```python
from build123d import *

# Parameters (mm, degrees)
SKETCH1_R           = 5
BOSS_EXTRUDE1_DEPTH = 150
SKETCH2_R           = 5
SKETCH2_R_2         = 4.8
CUT_EXTRUDE1_DEPTH  = 1.15
SKETCH3_R           = 5
SKETCH3_R_2         = 4.8
CUT_EXTRUDE2_DEPTH  = 1.15


with BuildPart() as part:
    # Sketch1 → Boss-Extrude1 (new, symmetric)
    with BuildSketch(Plane.XY):
        Circle(SKETCH1_R)
    extrude(amount=BOSS_EXTRUDE1_DEPTH, both=True)

    # Sketch2 → Cut-Extrude1 (cut)
    with BuildSketch(Plane.XY.offset(148)):
        Circle(SKETCH2_R)
        Circle(SKETCH2_R_2, mode=Mode.SUBTRACT)
    cut_extrude1 = extrude(amount=CUT_EXTRUDE1_DEPTH, mode=Mode.SUBTRACT)

    # Sketch3 → Cut-Extrude2 (cut)
    with BuildSketch(Plane.XY.offset(97.5)):
        Circle(SKETCH3_R)
        Circle(SKETCH3_R_2, mode=Mode.SUBTRACT)
    cut_extrude2 = extrude(amount=-CUT_EXTRUDE2_DEPTH, mode=Mode.SUBTRACT)

    # Mirror1: Cut-Extrude1, Cut-Extrude2 across plane
    add(cut_extrude1.mirror(Plane.XY), mode=Mode.SUBTRACT)
    add(cut_extrude2.mirror(Plane.XY), mode=Mode.SUBTRACT)


solid = part.part
```
The model under review builds one solid part; all positions refer to its coordinate system, in mm. A direction names the side the tool comes from. Coordinates: 2 decimals unless noted, no trailing zeros. Write each loop counter-clockwise with the first axis right and the second up, starting at its lowest first coordinate (ties: lowest second). Pieces come first, ordered by that corner, then holes. Notation, with made-up numbers: (49.25, 43.25) -> (59.25, 43.25) arc R8 ccw to (59.25, 56.25) -> close; hole circle Ø11 at (51, 34.5). An arc over 180 degrees is marked (long way). One line per item, written item: value. Start each with the question number.
Q1. Add section A-A, the plane z = 61. Give the boundary of the cut face in (x, y).
Q2. The part is to be moulded in two halves that separate along Z. For faces 1 (the face through (0, 0, -150)), 2 (the face through (-1.08, -4.88, 1.35)), 3 (the face through (2.58, 4.05, 148.57)), say which applies: +Z half, -Z half, draft (parallel to the pull), parting line (faces both ways), or undercut.
Q3. For faces 4 (the face through (-1.08, -4.88, -149.57)), 5 (the face through (2.58, 4.05, -148.57)), list the 3-axis set-ups (+Z, -Z, +X, -X, +Y, -Y) from which the entire face can be reached by the end or side of a thin tool; tool diameter is ignored.
Q4. To check wall thickness, follow probe 1 along Y at (x, z) = (-0.25, 137); probe 2 along Y at (x, z) = (-1.5, -91.5). State the ranges of each line that lie inside material, in increasing order.
Q5. Clearance check with flat-ended pins moving along their axes: P1, Ø2, axis at x = -1.5, z = -59, coming from the -Y side; P2, Ø6, axis at y = 0.5, z = 99.5, coming from the -X side; P3, Ø5, axis at x = -3.5, z = -77.5, coming from the +Y side; P4, Ø1.5, axis at y = -1.5, z = -104.5, coming from the -X side. State where each tip first meets the part, or that it passes through.
Response:
1. outline: circle Ø10 at (0, 0)
2. face 1: -Z half
2. face 2: draft
2. face 3: undercut
3. face 4: +Z, -Z
3. face 5: none
4. probe 1: -4.99 to 4.99
4. probe 2: -4.77 to 4.77
5. P1: y = -4.97
5. P2: x = -5
5. P3: y = 4.9
5. P4: x = -4.94
